from build123d import *

# Parameters (mm, degrees)
SKETCH1_W           = 38.5
SKETCH1_H           = 51.5
BOSS_EXTRUDE1_DEPTH = 40
SHELL1_T            = 4
SKETCH2_R           = 2.5
CUT_EXTRUDE3_DEPTH  = 4
FILLET2_R           = 1.5
SKETCH5_R           = 2
CUT_EXTRUDE4_DEPTH  = 56.005681525


with BuildPart() as part:
    # Sketch1 → Boss-Extrude1 (new body)
    with BuildSketch(Plane(origin=(0, 0, 0), x_dir=(1, 0, 0), z_dir=(0, 1, 0))):
        Rectangle(SKETCH1_W, SKETCH1_H)
    extrude(amount=BOSS_EXTRUDE1_DEPTH)

    # Shell1
    shell1_openings = [part.faces().sort_by_distance(p)[0] for p in [
        (0, 40, 0),
    ]]
    offset(amount=SHELL1_T, openings=shell1_openings, kind=Kind.INTERSECTION)

    # Sketch2 → Cut-Extrude3 (cut)
    with BuildSketch(Plane(origin=(0, 0, -29.75), x_dir=(-1, 0, 0), z_dir=(0, 0, -1))):
        with Locations(Location((0, 6, 0), (0, 0, 180))):
            Circle(SKETCH2_R)
    extrude(amount=-CUT_EXTRUDE3_DEPTH, mode=Mode.SUBTRACT)

    # Fillet2
    fillet2_edges = [part.edges().sort_by_distance(p)[0] for p in [
        (23.25, 40, 0),
        (0, 40, -29.75),
        (-19.25, 0, 0),
        (-19.25, 20, -25.75),
        (0, 0, 25.75),
        (-19.25, 20, 25.75),
        (19.25, 0, 0),
        (19.25, 20, 25.75),
        (0, 0, -25.75),
        (19.25, 20, -25.75),
        (-19.25, 40, 0),
        (0, 40, 25.75),
        (19.25, 40, 0),
        (0, 40, -25.75),
        (-23.25, 40, 0),
        (0, -4, -29.75),
        (23.25, -4, 0),
        (0, -4, 29.75),
        (-23.25, -4, 0),
        (-23.25, 18, -29.75),
        (23.25, 18, -29.75),
        (23.25, 18, 29.75),
        (-23.25, 18, 29.75),
        (0, 40, 29.75),
    ]]
    fillet(fillet2_edges, radius=FILLET2_R)

    # Sketch5 → Cut-Extrude4 (cut, through all)
    with BuildSketch(Plane(origin=(0, 0, 0), x_dir=(1, 0, 0), z_dir=(0, 1, 0))):
        with Locations(Location((-4.25, -16.25, 0), (0, 0, 270))):
            Circle(SKETCH5_R)
    extrude(amount=-CUT_EXTRUDE4_DEPTH, mode=Mode.SUBTRACT)


solid = part.part
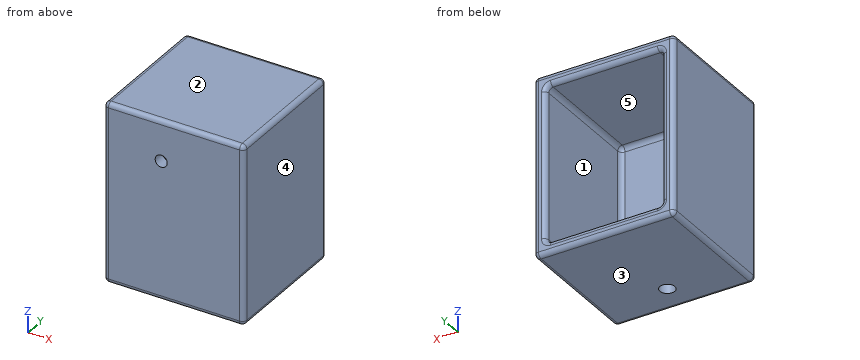
The listing builds one solid part. Answer for the finished solid, in the listing's coordinates (mm). Face numbers are marked on the shaded views. A direction names the side the tool comes from. Round coordinates to 2 decimals unless told otherwise and drop trailing zeros. Write each loop counter-clockwise with the first axis right and the second up, starting at its lowest first coordinate (ties: lowest second). Pieces come first, ordered by that corner, then holes. Notation, with made-up numbers: M 47.25,20 L 93.25,20 A20 ccw 93.25,28 Z; hole C 10.5,44.25 d2. An arc over 180 degrees is marked long. Write each question's results on one line, items separated by ' | '. Start each with the question number.
Item 1: Given pin 1 Ø1 at (x, z) = (3, 19.5) entering from +Y; pin 2 Ø4.5 at (x, y) = (0, 6) entering from -Z, each flat-ended and moving along its own axis, determine where each tip first touches the part or whether it passes through.
Item 2: Find section D-D on y = 6. Write down the section's boundary in (x, z).
Item 3: Straight lines are drawn through the part: probe 1 along Z at (x, y) = (-8.5, 3); probe 2 along X at (y, z) = (6, -27); probe 3 along X at (y, z) = (19, -15.5). For each, find the intervals that lie inside material, in ascending order.
Item 4: Find section A-A on x = 0. Write down the section's boundary in (y, z).
Item 5: Find section C-C on z = -16. Write down the section's boundary in (x, y).
Item 6: Which of the six approach directions +Z, -Z, +X, -X, +Y, -Y give full straight-line access (tool end or side, diameter ignored) to the marked faces 4 and 5?
Item 7: The mould has two halves that part along Z. Classify the marked faces 1, 2 and 3: +Z half, -Z half, draft (parallel to the pull), parting line (faces both ways), or undercut.
Item 8: Find section B-B on y = 12. Write down the section's boundary in (x, z).
Answer block:
1) pin 1: stops at y = 0 | pin 2: stops at z = 25.75
2) outline: M -23.25,-28.25 A1.5 ccw -21.75,-29.75 L -2.5,-29.75 L -2.5,-25.75 L -17.75,-25.75 A1.5 cw -19.25,-24.25 L -19.25,24.25 A1.5 cw -17.75,25.75 L 17.75,25.75 A1.5 cw 19.25,24.25 L 19.25,-24.25 A1.5 cw 17.75,-25.75 L 2.5,-25.75 L 2.5,-29.75 L 21.75,-29.75 A1.5 ccw 23.25,-28.25 L 23.25,28.25 A1.5 ccw 21.75,29.75 L -21.75,29.75 A1.5 ccw -23.25,28.25 Z
3) probe 1: z = -29.75 to -25.75, 25.75 to 29.75 | probe 2: x = -23.25 to -2.5, 2.5 to 23.25 | probe 3: x = -23.25 to -19.25, 19.25 to 23.25
4) outline: M -4,-28.25 A1.5 ccw -2.5,-29.75 L 3.5,-29.75 L 3.5,-25.75 L 1.5,-25.75 A1.5 cw 0,-24.25 L 0,24.25 A1.5 cw 1.5,25.75 L 38.5,25.75 A1.5 ccw 40,27.25 L 40,28.25 A1.5 ccw 38.5,29.75 L -2.5,29.75 A1.5 ccw -4,28.25 Z; M 8.5,-29.75 L 38.5,-29.75 A1.5 ccw 40,-28.25 L 40,-27.25 A1.5 ccw 38.5,-25.75 L 8.5,-25.75 Z
5) outline: M -23.25,-2.5 A1.5 ccw -21.75,-4 L 21.75,-4 A1.5 ccw 23.25,-2.5 L 23.25,38.5 A1.5 ccw 21.75,40 L 20.75,40 A1.5 ccw 19.25,38.5 L 19.25,1.5 A1.5 cw 17.75,0 L -17.75,0 A1.5 cw -19.25,1.5 L -19.25,38.5 A1.5 ccw -20.75,40 L -21.75,40 A1.5 ccw -23.25,38.5 Z
6) face 4: +Z, -Z, +X, +Y, -Y | face 5: +Y
7) face 1: undercut | face 2: +Z half | face 3: -Z half
8) outline: M -23.25,-28.25 A1.5 ccw -21.75,-29.75 L 21.75,-29.75 A1.5 ccw 23.25,-28.25 L 23.25,28.25 A1.5 ccw 21.75,29.75 L -21.75,29.75 A1.5 ccw -23.25,28.25 Z; hole M -19.25,-24.25 A1.5 ccw -17.75,-25.75 L 17.75,-25.75 A1.5 ccw 19.25,-24.25 L 19.25,24.25 A1.5 ccw 17.75,25.75 L -17.75,25.75 A1.5 ccw -19.25,24.25 Z
